```python
from build123d import *

# Parameters (mm, degrees)
SKETCH1_R             = 31
SKETCH1_R_2           = 28
BOSS_EXTRUDE1_DEPTH   = 14
SKETCH1_R_3           = 20.5
SKETCH1_R_4           = 17.5
BOSS_EXTRUDE1_2_DEPTH = 14
BOSS_EXTRUDE2_START   = 0.5
SKETCH1_3_R           = 28
SKETCH1_3_R_2         = 20.5
BOSS_EXTRUDE2_DEPTH   = 13


with BuildPart() as part:
    # Sketch1 → Boss-Extrude1 (new body)
    with BuildSketch(Plane(origin=(0, 0, 0), x_dir=(0, 1, 0), z_dir=(0, 0, 1))):
        Circle(SKETCH1_R)
        Circle(SKETCH1_R_2, mode=Mode.SUBTRACT)
    extrude(amount=BOSS_EXTRUDE1_DEPTH)



with BuildPart() as body_2:
    # Sketch1 → Boss-Extrude1 2 (new body)
    with BuildSketch(Plane(origin=(0, 0, 0), x_dir=(0, 1, 0), z_dir=(0, 0, 1))):
        Circle(SKETCH1_R_3)
        Circle(SKETCH1_R_4, mode=Mode.SUBTRACT)
    extrude(amount=BOSS_EXTRUDE1_2_DEPTH)


with BuildPart() as part_1:
    add(part.part)

    add(body_2.part)  # Boss-Extrude2 merges body 2
    # Sketch1<3> → Boss-Extrude2 (add)
    with BuildSketch(Plane(origin=(0, 0, 0), x_dir=(0, 1, 0), z_dir=(0, 0, 1)).offset(BOSS_EXTRUDE2_START)):
        Circle(SKETCH1_3_R)
        Circle(SKETCH1_3_R_2, mode=Mode.SUBTRACT)
    extrude(amount=BOSS_EXTRUDE2_DEPTH)


solid = part_1.part
```
Could you check a few things on this model? Use its own coordinates, in mm. A direction names the side the tool comes from. Round coordinates to 2 decimals unless told otherwise and drop trailing zeros. Loops run counter-clockwise (first coordinate to the right, second up) from the corner with the lowest first, then second, coordinate; pieces in that order, holes last. Notation, with made-up numbers: (15.25, 21) - (41.25, 21) arc R11 ccw to (41.25, 42) - close; hole circle Ø9 at (23, -34.5). An arc over 180 degrees is marked (long way). Answer as CSV lines item,"result".
1. For pin 1 Ø4 at (x, z) = (11, 4.5) entering from +Y; pin 2 Ø6 at (y, z) = (17, 3.5) entering from +X; pin 3 Ø1 at (x, z) = (1.5, 11) entering from -Y, each with a flat end and sliding along its axis, tell me the tip position at first contact or that it passes through.
Filled in:
pin 1,"stops at y = 29.66"
pin 2,"stops at x = 27.66"
pin 3,"stops at y = -30.98"
2. Please list where these lines run through material, in increasing order: line 1 along X through (y, z) = (0, 0.1); line 2 along Y through (x, z) = (0, 9.5). Write a range as [from, to].
Filled in:
line 1,"x = [-31, -28], [-20.5, -17.5], [17.5, 20.5], [28, 31]"
line 2,"y = [-31, -17.5], [17.5, 31]"
3. I want a section at C-C on z = 8. List the corners of the cut face in (x, y) for me, then the cut area to 3 significant figures.
Filled in:
outline,"circle Ø62 at (0, 0); hole circle Ø35 at (0, 0)"
area,"2,060 mm^2"
4. I want a section at D-D on y = 24.5. List the corners of the cut face in (x, z) for me.
Filled in:
outline,"(-18.99, 0) - (-13.56, 0) - (-13.56, 0.5) - (13.56, 0.5) - (13.56, 0) - (18.99, 0) - (18.99, 14) - (13.56, 14) - (13.56, 13.5) - (-13.56, 13.5) - (-13.56, 14) - (-18.99, 14) - close"
5. I want a section at A-A on x = 0. List the corners of the cut face in (y, z) for me.
Filled in:
outline,"(-31, 0) - (-28, 0) - (-28, 0.5) - (-20.5, 0.5) - (-20.5, 0) - (-17.5, 0) - (-17.5, 14) - (-20.5, 14) - (-20.5, 13.5) - (-28, 13.5) - (-28, 14) - (-31, 14) - close; (17.5, 0) - (20.5, 0) - (20.5, 0.5) - (28, 0.5) - (28, 0) - (31, 0) - (31, 14) - (28, 14) - (28, 13.5) - (20.5, 13.5) - (20.5, 14) - (17.5, 14) - close"
6. On a 3-axis mill with a long thin cutter (end or side, diameter ignored), from which of +Z, -Z, +X, -X, +Y, -Y can I reach the whole of each face in a straight line? I mean faces 4 (the face through (-9.2, 15.1, 0)), 5 (the face through (-15, -15, 0.5)), 6 (the face through (10.724, 25.865, 13.746)). Say none if no direction works.
Filled in:
face 4,"-Z, +X, -X, +Y, -Y"
face 5,"-Z"
face 6,"+Z"
7. We'd pull the mould along X, two halves only. Please class faces 1 (the face through (-9.2, 15.1, 14)), 2 (the face through (20.013, -4.444, 0.246)), 3 (the face through (-30.736, -4.036, 6.902)): +X half, -X half, draft (parallel to the pull), parting line (faces both ways), or undercut.
Filled in:
face 1,"draft"
face 2,"undercut"
face 3,"parting line"
